from build123d import *

# Parameters (mm, degrees)
EXTRUSION1_DEPTH = 39
ESQUISSE2_R      = 5.5
EXTRUSION2_DEPTH = 10
ESQUISSE3_R      = 1.5
EXTRUSION3_DEPTH = 47.864006287


with BuildPart() as part:
    # Esquisse1 → Extrusion1 (new body)
    with BuildSketch(Plane.XY):
        Polygon((-16.636265327, 16.590210526), (-16.636265327, -3.409789474), (3.363734673, -3.409789474), (3.363734673, 16.590210526), (1.863734673, 16.590210526), (1.863734673, -1.909789474), (-15.136265327, -1.909789474), (-15.136265327, 16.590210526), align=None)
    extrude(amount=EXTRUSION1_DEPTH)

    # Esquisse2 → Extrusion2 (cut)
    with BuildSketch(Plane(origin=(3.363734673, 0, 0), x_dir=(0, 0, -1), z_dir=(1, 0, 0))):
        with Locations((-19.5, 16.590210526)):
            Circle(ESQUISSE2_R)
    extrude(amount=-EXTRUSION2_DEPTH, mode=Mode.SUBTRACT)

    # Esquisse3 → Extrusion3 (cut, through all)
    with BuildSketch(Plane.ZY.offset(16.636265327)):
        with Locations(Location((3.5, 0.590210526, 0), (0, 0, 270))):
            Circle(ESQUISSE3_R)
        with Locations(Location((35.5, 0.590210526, 0), (0, 0, 270))):
            Circle(ESQUISSE3_R)
    extrude(amount=-EXTRUSION3_DEPTH, mode=Mode.SUBTRACT)


solid = part.part
Could you check a few things on this model? Use its own coordinates, in mm. A direction names the side the tool comes from. Give positions to 0.01 mm unless a question says otherwise; leave off trailing zeros. Write each loop counter-clockwise with the first axis right and the second up, starting at its lowest first coordinate (ties: lowest second). Pieces come first, ordered by that corner, then holes. Notation, with made-up numbers: (-8.5, 3.5) -> (1.5, 3.5) arc R12 ccw to (1.5, 8.5) -> close; hole circle Ø6 at (-19, 32). An arc over 180 degrees is marked (long way). Write each question's results on one line, items separated by ' | '. Start each with the question number.
Q1. We'd pull the mould along Z, two halves only. Please class faces 4 (the face through (3, 16.59, 7)), 5 (the face through (-6.7, -2.3, 39)), 6 (the face through (2.603, 0.915, 2.036)), 7 (the face through (-6.7, -2.3, 0)): +Z half, -Z half, draft (parallel to the pull), parting line (faces both ways), or undercut.
Q2. I need wall thicknesses on probe 1 along X at (y, z) = (3.75, 24); probe 2 along Y at (x, z) = (-12.25, 18). Which ranges of each line are inside material? Lowest first, please.
Q3. I'm going to push flat-ended pins straight in: pin 1 Ø1.8 at (y, z) = (0.59, 3.5) entering from +X; pin 2 Ø1 at (x, z) = (-10.5, 29) entering from +Y. Where does each tip first touch, or does it pass through?
Q4. Suppose I cut it at A-A, the plane y = 3.75. List the corners of the cut face in (x, z) for me.
Q5. Suppose I cut it at B-B, the plane z = 3.5. List the corners of the cut face in (x, y) for me, and give its area (3 significant figures).
Q6. Which directions (+Z, -Z, +X, -X, +Y, -Y) give clear straight access to the entire face, cutting with the end or side of a thin tool? Please do faces 1 (the face through (1.864, 7, 19)), 2 (the face through (2.62, 11.09, 19.62)), 3 (the face through (-7, -3.41, 19)).
Q7. Suppose I cut it at D-D, the plane z = 32.5. List the corners of the cut face in (x, y) for me.
Q8. Suppose I cut it at C-C, the plane y = -0.25. List the corners of the cut face in (x, z) for me.
Outcome:
1) face 4: draft | face 5: +Z half | face 6: undercut | face 7: -Z half
2) probe 1: -16.64 to -15.14, 1.86 to 3.36 | probe 2: -3.41 to -1.91
3) pin 1: through | pin 2: y = -1.91
4) outline: (-16.64, 0) -> (-15.14, 0) -> (-15.14, 39) -> (-16.64, 39) -> close; (1.86, 0) -> (3.36, 0) -> (3.36, 39) -> (1.86, 39) -> close
5) outline: (-16.64, -3.41) -> (3.36, -3.41) -> (3.36, -0.91) -> (1.86, -0.91) -> (1.86, -1.91) -> (-15.14, -1.91) -> (-15.14, -0.91) -> (-16.64, -0.91) -> close; (-16.64, 2.09) -> (-15.14, 2.09) -> (-15.14, 16.59) -> (-16.64, 16.59) -> close; (1.86, 2.09) -> (3.36, 2.09) -> (3.36, 16.59) -> (1.86, 16.59) -> close | area: 76.5 mm2
6) face 1: +Z, -Z, +Y | face 2: +X, +Y | face 3: +Z, -Z, +X, -X, -Y
7) outline: (-16.64, -3.41) -> (3.36, -3.41) -> (3.36, 16.59) -> (1.86, 16.59) -> (1.86, -1.91) -> (-15.14, -1.91) -> (-15.14, 16.59) -> (-16.64, 16.59) -> close
8) outline: (-16.64, 0) -> (-15.14, 0) -> (-15.14, 2.26) -> (-16.64, 2.26) -> close; (-16.64, 4.74) -> (-15.14, 4.74) -> (-15.14, 34.26) -> (-16.64, 34.26) -> close; (-16.64, 36.74) -> (-15.14, 36.74) -> (-15.14, 39) -> (-16.64, 39) -> close; (1.86, 0) -> (3.36, 0) -> (3.36, 2.26) -> (1.86, 2.26) -> close; (1.86, 4.74) -> (3.36, 4.74) -> (3.36, 34.26) -> (1.86, 34.26) -> close; (1.86, 36.74) -> (3.36, 36.74) -> (3.36, 39) -> (1.86, 39) -> close
